```python
from build123d import *

# Parameters (mm, degrees)
SKETCH1_R               = 9
BOSS_EXTRUDE1_DEPTH     = 25
SKETCH2_R               = 6
BOSS_EXTRUDE2_DEPTH     = 40
CUT_EXTRUDE2_DEPTH      = 42.976183724
CUT_EXTRUDE2_DEPTH_BACK = 42.976183724
SKETCH3_R               = 3


with BuildPart() as part:
    # Sketch1 → Boss-Extrude1 (new, symmetric)
    with BuildSketch(Plane.XY):
        Circle(SKETCH1_R)
    extrude(amount=BOSS_EXTRUDE1_DEPTH, both=True)

    # Sketch2 → Boss-Extrude2 (add, symmetric)
    with BuildSketch(Plane.XY):
        Circle(SKETCH2_R)
    extrude(amount=BOSS_EXTRUDE2_DEPTH, both=True)

    # Sketch3 → Cut-Extrude2 (cut, two sides: drawn at the far end of the back side and taken through both)
    with BuildSketch(Plane(origin=(0, 0, 0), x_dir=(0, 0, -1), z_dir=(1, 0, 0)).offset(-CUT_EXTRUDE2_DEPTH_BACK)):
        Circle(SKETCH3_R)
    extrude(amount=CUT_EXTRUDE2_DEPTH + CUT_EXTRUDE2_DEPTH_BACK, mode=Mode.SUBTRACT)


solid = part.part
```
CAD build for the part. Positions are in the model's coordinates, mm. A direction names the side the tool comes from. Coordinates: 2 decimals unless noted, no trailing zeros. Write each loop counter-clockwise with the first axis right and the second up, starting at its lowest first coordinate (ties: lowest second). Pieces come first, ordered by that corner, then holes.
(1) 3-axis set-ups, long thin cutter, end or side, ignore diameter. For faces 1 (the face through (2, -6, 25)), 2 (the face through (-1.951, -8.786, 0.35)), 3 (the face through (2, -6, -25)): which of +Z, -Z, +X, -X, +Y, -Y reach the whole face in a straight line?
(2) Cut at A-A, the plane y = 0. List the corners of the cut face in (x, z), and give its area (3 significant figures).
(3) Flat gauge pins, fed straight in: pin 1 (6 mm diameter, centred on y = 6.5, z = 31.5, fed in from +X); pin 2 (10 mm diameter, centred on x = 5.5, z = 24.5, fed in from +Y); pin 3 (2 mm diameter, centred on x = -3, z = 24.5, fed in from +Y); pin 4 (5 mm diameter, centred on y = 0, z = 0, fed in from +X). Where does each tip first touch, or does it go through?
(4) Cut at D-D, the plane z = 13. List the corners of the cut face in (x, y), and give its area (3 significant figures).
(5) Two-plate mould, pull along Y, no slides. Class faces 4 (the face through (-6, 0, -32)), 5 (the face through (0, 0, -40)), 6 (the face through (0, 0, 3)): +Y half, -Y half, draft (parallel to the pull), parting line (faces both ways), or undercut.
(6) Drill centre lines: probe 1 along Z at (x, y) = (-2.25, 0); probe 2 along Z at (x, y) = (-1.75, 7.75); probe 3 along Y at (x, z) = (4.75, 0). Where is each one in solid material? Low to high.
(7) Cut at C-C, the plane y = 4.5. List the corners of the cut face in (x, z), and give its area (3 significant figures).
(8) Cut at B-B, the plane x = 0. List the corners of the cut face in (y, z).
Geometry says:
1. face 1: +Z
1. face 2: +Z, -Z
1. face 3: -Z
2. outline: (-9, -25) - (-6, -25) - (-6, -40) - (6, -40) - (6, -25) - (9, -25) - (9, -3) - (-9, -3) - close; (-9, 3) - (9, 3) - (9, 25) - (6, 25) - (6, 40) - (-6, 40) - (-6, 25) - (-9, 25) - close
2. area: 1,150 mm2
3. pin 1: stops at x = 4.87
3. pin 2: stops at y = 8.99
3. pin 3: stops at y = 8.77
3. pin 4: passes through
4. outline: circle Ø18 at (0, 0)
4. area: 254 mm2
5. face 4: parting line
5. face 5: draft
5. face 6: undercut
6. probe 1: z = -40 to -3, 3 to 40
6. probe 2: z = -25 to 25
6. probe 3: y = -7.64 to -3, 3 to 7.64
7. outline: (-7.79, -25) - (-3.97, -25) - (-3.97, -40) - (3.97, -40) - (3.97, -25) - (7.79, -25) - (7.79, 25) - (3.97, 25) - (3.97, 40) - (-3.97, 40) - (-3.97, 25) - (-7.79, 25) - close
7. area: 1,020 mm2
8. outline: (-9, -25) - (-6, -25) - (-6, -40) - (6, -40) - (6, -25) - (9, -25) - (9, 25) - (6, 25) - (6, 40) - (-6, 40) - (-6, 25) - (-9, 25) - close; hole circle Ø6 at (0, 0)
